Autodesk Inventor part; units mm, degrees
ref_plane "Work Plane1" through (0, 0, 6.35) normal (0, 0, 1) x (1, 0, 0)
ref_plane "YZ Plane" through (0, 0, 0) normal (1, 0, 0) x (0, 1, 0)
ref_plane "XZ Plane" through (0, 0, 0) normal (0, 1, 0) x (-1, 0, 0)
sketch "Sketch1" plane through (0, 0, 0) normal (0, 0, 1) x (1, 0, 0)
  circle A0 centre (0, 0) radius 7.1437
  dimension "d0" = 14.2875
extrude "Extrusion1" add sketch "Sketch1" along normal blind 5.3975
ref_plane "Work Plane1" through (0, 0, 6.35) normal (0, 0, 1) x (1, 0, 0)
sketch "Sketch6" plane through (0, 0, 5.3975) normal (0, 0, 1) x (1, 0, 0)
  circle A0 centre (0, 0) radius 2.4892
  dimension "d28" = 4.9784
extrude "Extrusion3" cut sketch "Sketch6" against normal through all
sketch "Sketch7" plane through (0, 0, 5.3975) normal (0, 0, 1) x (1, 0, 0)
  circle A0 centre (0, 0) radius 4.7625
  circle A1 centre (0, 0) radius 2.4892
  dimension "d31" = 9.525
  dimension "d32" = 4.9784
extrude "Extrusion4" add sketch "Sketch7" along normal blind 5.5563
sketch "Sketch8" plane through (0, 0, 0) normal (0, 0, -1) x (-1, 0, 0)
  circle A0 centre (0, 0) radius 2.4892
  circle A1 centre (0, 0) radius 4.7625
extrude "Extrusion5" add sketch "Sketch8" along normal blind 5.5563
ref_plane "Work Plane2" through (0, 0, 2.6987) normal (0, 0, 1) x (1, 0, 0)
properties part number "RollerSpacer2(Bearing)"
Source: CAD feature listing. Evaluate the final solid. Frame: model axes, mm. A direction names the side the tool comes from. Coordinates: 2 decimals unless noted, no trailing zeros. Write each loop counter-clockwise with the first axis right and the second up, starting at its lowest first coordinate (ties: lowest second). Pieces come first, ordered by that corner, then holes. Notation, with made-up numbers: (38, -5.75) -> (88, -5.75) arc R7 ccw to (88, 7.25) -> close; hole circle Ø5 at (-20.5, 18.5). An arc over 180 degrees is marked (long way). Return JSON: item names as keys, results as strings. Group by question number.
1) Mould query, pull axis Y, two halves, no side actions, for faces 1 (the face through (6.814, -2.146, 2.661)), 2 (the face through (0.164, 2.484, 2.814)), 3 (the face through (-2, -2, -5.556)). Classes: +Y half, -Y half, draft (parallel to the pull), parting line (faces both ways), or undercut.
2) Section query A-A, the plane y = 0. Return loops of the section in (x, z).
3) Contact query for flat-ended pins moving along their axis: P1, Ø4, axis at x = -2, z = 8.5, coming from the +Y side; P2, Ø1.5, axis at x = -1.5, z = 2, coming from the +Y side; P3, Ø3, axis at y = -4.5, z = 3, coming from the -X side. Output: stop coordinate, or through.
4) Set-up query: faces 4 (the face through (2, -2, 10.954)), 5 (the face through (3.78, 2.9, -2.74)), 6 (the face through (5, -1, 5.398)). Return all of +Z, -Z, +X, -X, +Y, -Y with unobstructed straight access to the full face (end or side cutting, diameter ignored); none if empty.
5) Section query C-C, the plane z = 10.25. Return loops of the section in (x, y) (1 decimal).
6) Ray query, line 1 along Y through (x, z) = (0, 6); line 2 along Y through (x, z) = (0, 0.25); line 3 along Z through (x, y) = (4.75, 4.5). Return the intervals inside material, ascending.
7) Section query D-D, the plane x = -3.5. Return loops of the section in (y, z), plus the area to 3 significant figures.
From the geometry:
{
 "1": {"face 1": "parting line", "face 2": "undercut", "face 3": "draft"},
 "2": {"outline": "(-7.14, 0) -> (-4.76, 0) -> (-4.76, -5.56) -> (-2.49, -5.56) -> (-2.49, 10.95) -> (-4.76, 10.95) -> (-4.76, 5.4) -> (-7.14, 5.4) -> close; (2.49, -5.56) -> (4.76, -5.56) -> (4.76, 0) -> (7.14, 0) -> (7.14, 5.4) -> (4.76, 5.4) -> (4.76, 10.95) -> (2.49, 10.95) -> close"},
 "3": {"P1": "y = 4.76", "P2": "y = 7.1", "P3": "x = -6.48"},
 "4": {"face 4": "+Z, +X, -X, +Y, -Y", "face 5": "-Z", "face 6": "+Z"},
 "5": {"outline": "circle Ø9.5 at (0, 0); hole circle Ø5 at (0, 0)"},
 "6": {"line 1": "-4.76 to -2.49, 2.49 to 4.76", "line 2": "-7.14 to -2.49, 2.49 to 7.14", "line 3": "0 to 5.4"},
 "7": {"outline": "(-6.23, 0) -> (-3.23, 0) -> (-3.23, -5.56) -> (3.23, -5.56) -> (3.23, 0) -> (6.23, 0) -> (6.23, 5.4) -> (3.23, 5.4) -> (3.23, 10.95) -> (-3.23, 10.95) -> (-3.23, 5.4) -> (-6.23, 5.4) -> close", "area": "139 mm²"}
}
